CAD build for the part. Positions are in the model's coordinates, mm. A direction names the side the tool comes from. Give positions to 0.01 mm unless a question says otherwise; leave off trailing zeros. Loops run counter-clockwise (first coordinate to the right, second up) from the corner with the lowest first, then second, coordinate; pieces in that order, holes last. Notation, with made-up numbers: (12.5, 30) -> (29.5, 30) arc R14 cw to (29.5, 55) -> close; hole circle Ø5 at (-19, -24.5). An arc over 180 degrees is marked (long way). Use one line per item in the form item = value.
```python
from build123d import *

# Parameters (mm, degrees)
F0_R     = 4.9
F0_R_2   = 3.95
F1_DEPTH = 3
F0_R_3   = 2
F2_DEPTH = 8.4
F3_R     = 0.25


with BuildPart() as f1:
    # F0 (on Top) → F1 (new body)
    with BuildSketch(Plane.XY):
        Circle(F0_R)
        Circle(F0_R_2, mode=Mode.SUBTRACT)
    extrude(amount=F1_DEPTH)

    # F0 (on Top) → F2 (join)
    with BuildSketch(Plane.XY):
        Circle(F0_R_2)
        Circle(F0_R_3, mode=Mode.SUBTRACT)
    extrude(amount=F2_DEPTH)

    # F3
    f3_edges = [f1.edges().sort_by_distance(p)[0] for p in [
        (-2, 0, 8.4),
    ]]
    fillet(f3_edges, radius=F3_R)


solid = f1.part
```
1. Drop flat-ended pins along their axis: P1, Ø1, axis at x = 1, z = 1.5, coming from the +Y side; P2, Ø1.5, axis at y = -0.5, z = 4, coming from the +X side; P3, Ø1.5, axis at y = 2.5, z = 2, coming from the -X side. Give the stop position or say it passes through.
Result sheet:
P1 = 4.87
P2 = 3.95
P3 = -4.58
2. Drill centre lines: line 1 (Y direction, x = 0, z = 6); line 2 (Y direction, x = 0, z = 2); line 3 (Z direction, x = 4, y = -0.5). Where is each one in solid material? Low to high.
Result sheet:
line_1 = -3.95 to -2, 2 to 3.95
line_2 = -4.9 to -2, 2 to 4.9
line_3 = 0 to 3
3. Cut at A-A, the plane x = 0. Write the cut outline in (y, z), then the cut area to 3 significant figures.
Result sheet:
outline = (-4.9, 0) -> (-2, 0) -> (-2, 8.15) arc R0.25 ccw to (-2.25, 8.4) -> (-3.95, 8.4) -> (-3.95, 3) -> (-4.9, 3) -> close; (2, 0) -> (4.9, 0) -> (4.9, 3) -> (3.95, 3) -> (3.95, 8.4) -> (2.25, 8.4) arc R0.25 ccw to (2, 8.15) -> close
area = 38.4 mm^2
4. Mould opens along Y. For faces 1 (the cylindrical face through (-1.062, -4.783, 1.479)), 2 (the cylindrical face through (0, -2, 4)), 3 (the flat face through (2, -1, 0)) say: pulls with the +Y half, pulls with the -Y half, needs draft (parallel to the pull), parting line crosses it, or undercut.
Result sheet:
face_1 = parting line crosses it
face_2 = undercut
face_3 = needs draft
5. Tool access for faces 4 (the flat face through (2, -2, 8.4)), 5 (the cylindrical face through (-3.135, -2.404, 5.662)): list every direction of +Z, -Z, +X, -X, +Y, -Y with a clear straight run to the whole face (end or side of a thin tool).
Result sheet:
face_4 = +Z, +X, -X, +Y, -Y
face_5 = +Z
6. Cut at C-C, the plane z = 4.75. Write the cut outline in (x, y).
Result sheet:
outline = circle Ø7.9 at (0, 0); hole circle Ø4 at (0, 0)
7. Cut at D-D, the plane x = 3.25. Write the cut outline in (y, z) (3 decimals), then the cut area to 3 significant figures.
Result sheet:
outline = (-3.667, 0) -> (3.667, 0) -> (3.667, 3) -> (2.245, 3) -> (2.245, 8.4) -> (-2.245, 8.4) -> (-2.245, 3) -> (-3.667, 3) -> close
area = 46.2 mm^2
